Model file for the job. Use its own axes, mm. A direction names the side the tool comes from. Round coordinates to 2 decimals unless told otherwise and drop trailing zeros. Loops run counter-clockwise (first coordinate to the right, second up) from the corner with the lowest first, then second, coordinate; pieces in that order, holes last. Notation, with made-up numbers: (-33.75, -21) -> (13.25, -21) arc R6 ccw to (13.25, -12) -> close; hole circle Ø7 at (1.5, -36). An arc over 180 degrees is marked (long way). Use a Markdown table: item, result. Add a question column.
Autodesk Inventor part; units mm, degrees
ref_plane "YZ Plane" through (0, 0, 0) normal (1, 0, 0) x (0, 1, 0)
ref_plane "XZ Plane" through (0, 0, 0) normal (0, 1, 0) x (-1, 0, 0)
ref_plane "XY Plane" through (0, 0, 0) normal (0, 0, 1) x (1, 0, 0)
sketch "Sketch1" plane through (0, 0, 0) normal (0, 1, 0) x (-1, 0, 0)
  arc A0 (-0.3814, 2.9757) -> (-3, 0) centre (0, 0) ccw
  arc A1 (-0.3814, 2.9757) -> (0, 75) centre (-5, 39.0133) ccw
  line L0 (-105, 0) -> (0, 0) construction
  line L1 (-3, 0) -> (-105, 0) construction
  arc A2 (-3, 0) -> (-0.3814, -2.9757) centre (0, 0) ccw
  arc A3 (-1.6619, -2.4976) -> (97.0992, -0.9275) centre (46.5785, 70) ccw
  arc A4 (102.9008, -9.0725) -> (97.0992, -0.9275) centre (100, -5) ccw
  line L2 (0, 0) -> (100, 0) construction
  arc A5 (5.6849, -18.0476) -> (102.9008, -9.0725) centre (46.5785, 70) ccw
  line L3 (0, 75) -> (0, 0) construction
  line L4 (0, 0) -> (0, -15.1769) construction
  line L5 (0, 0) -> (-105, 0) construction
  line L6 (0, 75) -> (-105, 75)
  line L7 (-105, 75) -> (-105, -25)
  line L8 (0, -21.6754) -> (0, -21)
  line L9 (-4, -25) -> (-105, -25)
  arc A6 (5.6849, -18.0476) -> (0, -21.6754) centre (4, -21.6754) ccw
  arc A7 (-4, -25) -> (0, -21) centre (-4, -21) ccw
  circle A8 centre (-5, 35) radius 11
  point P0 (-5, -39.0133)
  point P1 (0, -25)
  dimension "d0" = 6
  dimension "d13" = 5
  dimension "d47" = 10
  dimension "d48" = 100
  dimension "d49" = 100
  dimension "d68" = 70
  dimension "d71" = 0
  dimension "d73" = 25
  dimension "d75" = 105
  dimension "d76" = 4
  dimension "d77" = 4
  dimension "d101" = 22
  dimension "d102" = 5
  dimension "d103" = 35
  dimension "d108" = 75
extrude "Extrusion1" add sketch "Sketch1" along normal blind 2
sketch "Szkic5" plane through (0, 2, 0) normal (0, 1, 0) x (1, 0, 0)
  circle A0 centre (12.5, -67.5) radius 2.1
  circle A1 centre (97.5, -67.5) radius 2.1
  line L0 (97.5, -67.5) -> (97.5, 52.5) construction
  line L1 (12.5, -67.5) -> (97.5, -67.5) construction
  line L2 (0, -75) -> (105, -75) construction
  line L3 (105, -75) -> (105, 25) construction
  line L4 (105, 25) -> (4, 25) construction
  line L5 (0, 21) -> (0, 21.6754) construction
  circle A2 centre (97.5, 20) radius 2.1
  circle A3 centre (12.5, 20) radius 2.1
  line L6 (12.5, 20) -> (97.5, 20) construction
  point P0 (0, 0)
  dimension "d84" = 7.5
  dimension "d85" = 7.5
  dimension "d89" = 85
  dimension "d106" = 87.5
  dimension "d107" = 85
  dimension "d109" = 4.2
extrude "Wyciągnięcie proste4" cut sketch "Szkic5" against normal up to surface (2 mm away)
sketch "Szkic6" plane through (0, 2, 0) normal (0, 1, 0) x (1, 0, 0)
  line L0 (105, -55) -> (100.9, -55)
  line L1 (100.9, -55) -> (100.9, -40)
  line L2 (100.9, -40) -> (105, -40)
  line L3 (105, -40) -> (105, -55)
  line L4 (105, -10) -> (100.9, -10)
  line L5 (100.9, -10) -> (100.9, 5)
  line L6 (100.9, 5) -> (105, 5)
  line L7 (105, 5) -> (105, -10)
  line L8 (100.9, -40) -> (100.9, -10) construction
  line L9 (105, -75) -> (105, 25) construction
  line L10 (100.9, -25) -> (105, -25) construction
  point P0 (0, 0)
  dimension "d92" = 15
  dimension "d94" = 30
  dimension "d134" = 4.1
extrude "Wyciągnięcie proste5" cut sketch "Szkic6" against normal up to surface (2 mm away)
sketch "Sketch9" plane through (0, 2, 0) normal (0, 1, 0) x (1, 0, 0)
  line L0 (-11.5, -35) -> (21.5, -35) construction
  circle A0 centre (-11.5, -35) radius 1.6
  circle A1 centre (21.5, -35) radius 1.6
  circle A2 centre (5, -35) radius 11 construction
  point P0 (0, 0)
  dimension "d110" = 33
  dimension "d111" = 3.2
extrude "Extrusion6" cut sketch "Sketch9" against normal through all
fillet "Fillet1" radius 5 1 edges at (105, 1, -25)
sketch "Sketch10" plane through (0, 2, 0) normal (0, 1, 0) x (1, 0, 0)
  circle A0 centre (6, 12.5) radius 1.75
  circle A1 centre (34, 12.5) radius 1.75
  line L0 (6, 12.5) -> (34, 12.5) construction
  line L1 (100, 25) -> (4, 25) construction
  point P0 (0, 0)
  dimension "d115" = 3.5
  dimension "d116" = 28
  dimension "d117" = 12.5
  dimension "d118" = 6
extrude "Extrusion7" cut sketch "Sketch10" against normal through all
sketch "Sketch11" plane through (0, 2, 0) normal (0, 1, 0) x (1, 0, 0)
  line L0 (93.5, -75) -> (51.5, -75)
  line L1 (51.5, -75) -> (51.5, -18)
  line L2 (51.5, -18) -> (93.5, -18)
  line L3 (93.5, -18) -> (93.5, -75)
  line L4 (0, -75) -> (105, -75) construction
  point P0 (0, 0)
  point P1 (100, -75)
  dimension "d121" = 42
  dimension "d122" = 57
  dimension "d123" = 51.5
extrude "Extrusion8" cut sketch "Sketch11" against normal through all
sketch "Sketch12" plane through (0, 2, 0) normal (0, 1, 0) x (1, 0, 0)
  line L0 (93.5, -75) -> (105, -75)
  line L1 (93.5, -75) -> (93.5, -90.5)
  line L2 (93.5, -90.5) -> (51.5, -90.5)
  line L3 (0, -75) -> (51.5, -75)
  line L4 (51.5, -90.5) -> (51.5, -75)
  line L5 (93.5, -75) -> (105, -75)
  line L6 (105, -75) -> (105, -98.5)
  line L7 (105, -98.5) -> (43.5, -98.5)
  line L8 (43.5, -98.5) -> (43.5, -75)
  point P0 (0, 0)
  dimension "d126" = 15.5
  dimension "d127" = 8
  dimension "d128" = 8
extrude "Extrusion9" add sketch "Sketch12" against normal up to surface (2 mm away)
fillet "Fillet2" radius 5 3 edges at (43.5, 1, 75) (43.5, 1, 98.5) (105, 1, 98.5)
fillet "Fillet3" radius 1 4 edges at (51.5, 1, 18) (93.5, 1, 18) (93.5, 1, 90.5) (51.5, 1, 90.5)
fillet "Fillet4" radius 2 4 edges at (105, 1, 55) (105, 1, 40) (105, 1, 10) (105, 1, -5)
sketch "Sketch13" plane through (0, 2, 0) normal (0, 1, 0) x (1, 0, 0)
  line L0 (99.25, -77.5) -> (99.25, -93.5) construction
  line L1 (93.5, -19) -> (93.5, -89.5) construction
  line L2 (93.5, -89.5) -> (105, -89.5) construction
  line L3 (105, -93.5) -> (105, -57) construction
  point P0 (0, 0)
  point P1 (99.25, -89.5)
  dimension "d137" = 12
  dimension "d138" = 4
hole "Hole1" at (99.25, 2, 77.5) at (99.25, 2, 93.5) direction (0, -1, 0) diameter 3.2 end through all
sketch "Sketch14" plane through (0, 2, 0) normal (0, 1, 0) x (1, 0, 0)
  arc A0 (1.6619, 2.4976) -> (-97.0992, 0.9275) centre (-46.5785, -70) ccw construction
  arc A1 (-102.9008, 9.0725) -> (-97.0992, 0.9275) centre (-100, 5) ccw
  arc A2 (13.245, 0) -> (-100, 5) centre (-46.5785, -70) ccw construction
  line L0 (0, 0) -> (13.245, 0) construction
  line L1 (-46.5785, -70) -> (-100, 5) construction
  line L2 (24.9599, 21) -> (84.9599, 21) construction
  circle A3 centre (12.5, 20) radius 2.1
  circle A4 centre (97.5, 20) radius 2.1
  line L3 (100, 25) -> (4, 25)
  line L4 (0, -70) -> (38.5, -70) construction
  arc A5 (43.5, -80) -> (38.5, -75) centre (38.5, -80) ccw
  line L5 (38.5, -70) -> (38.5, -75) construction
  line L6 (0, -75) -> (0, -70) construction
  line L7 (0, -75) -> (38.5, -75)
  arc A6 (100, -98.5) -> (105, -93.5) centre (100, -93.5) ccw
  line L8 (48.5, -93.5) -> (100, -93.5) construction
  arc A7 (43.5, -93.5) -> (48.5, -98.5) centre (48.5, -93.5) ccw construction
  arc A8 (100, -98.5) -> (105, -93.5) centre (100, -93.5) ccw construction
  point P0 (54.9599, 21)
  point P1 (74.25, -93.5)
  point P2 (-78.7683, 16.2709)
  point P3 (-78.7683, 16.2709)
  point P4 (-78.7683, 16.2709)
  point P5 (-55.3429, 21.6626)
  point P6 (-55.3429, 21.6626)
  point P7 (-55.3429, 21.6626)
  point P8 (-31.3202, 20.8077)
  point P9 (-31.3202, 20.8077)
  point P10 (-31.3202, 20.8077)
  point P11 (-8.3374, 13.7643)
  point P12 (-8.3374, 13.7643)
  point P13 (-8.3374, 13.7643)
  dimension "d150" = 60
  dimension "d151" = 12.5
  dimension "d152" = 4
  dimension "d153" = 5
  dimension "d156" = 60
hole "Hole2" at (-100, 2, -5) at (24.9599, 2, -21) at (54.9599, 2, -21) at (84.9599, 2, -21) at (0, 2, 70) at (38.5, 2, 70) at (48.5, 2, 93.5) at (74.25, 2, 93.5) at (-78.7683, 2, -16.2709) at (-55.3429, 2, -21.6626) at (-31.3202, 2, -20.8077) at (-8.3374, 2, -13.7643) direction (0, -1, 0) diameter 3.2 end through all
sketch "Sketch15" plane through (0, 2, 0) normal (0, 1, 0) x (1, 0, 0)
  line L0 (30, -40) -> (31.5, -40)
  line L1 (31.5, -40) -> (31.5, -51)
  line L2 (31.5, -51) -> (30, -51)
  line L3 (30, -51) -> (30, -40)
  line L4 (41.5, -40) -> (43, -40)
  line L5 (43, -40) -> (43, -51)
  line L6 (43, -51) -> (41.5, -51)
  line L7 (41.5, -51) -> (41.5, -40)
  point P0 (0, 0)
  dimension "d165" = 1.5
  dimension "d166" = 11
  dimension "d167" = 10
  dimension "d168" = 40
  dimension "d169" = 30
extrude "Extrusion10" cut sketch "Sketch15" against normal through all
sketch "Sketch16" plane through (0, 2, 0) normal (0, 1, 0) x (1, 0, 0)
  line L0 (43, -40) -> (43, -51)
  line L1 (43, -51) -> (41.5, -51)
  line L2 (41.5, -51) -> (41.5, -40)
  line L3 (41.5, -40) -> (43, -40)
  line L4 (31.5, -40) -> (31.5, -51)
  line L5 (31.5, -51) -> (30, -51)
  line L6 (30, -51) -> (30, -40)
  line L7 (30, -40) -> (31.5, -40)
  circle A0 centre (-31.3202, 20.8077) radius 1.6
  circle A1 centre (-78.7683, 16.2709) radius 1.6
  circle A2 centre (48.5, -93.5) radius 1.6
  circle A3 centre (0, -70) radius 1.6
  circle A4 centre (54.9599, 21) radius 1.6
  circle A5 centre (-100, 5) radius 1.6
  circle A6 centre (24.9599, 21) radius 1.6
  circle A7 centre (84.9599, 21) radius 1.6
  circle A8 centre (38.5, -70) radius 1.6
  circle A9 centre (74.25, -93.5) radius 1.6
  circle A10 centre (-55.3429, 21.6626) radius 1.6
  circle A11 centre (-8.3374, 13.7643) radius 1.6
  circle A12 centre (99.25, -77.5) radius 1.6
  circle A13 centre (99.25, -93.5) radius 1.6
  line L8 (51.5, -89.5) -> (51.5, -19)
  arc A14 (52.5, -18) -> (51.5, -19) centre (52.5, -19) ccw
  line L9 (52.5, -18) -> (92.5, -18)
  arc A15 (93.5, -19) -> (92.5, -18) centre (92.5, -19) ccw
  line L10 (93.5, -19) -> (93.5, -89.5)
  arc A16 (92.5, -90.5) -> (93.5, -89.5) centre (92.5, -89.5) ccw
  line L11 (92.5, -90.5) -> (52.5, -90.5)
  arc A17 (51.5, -89.5) -> (52.5, -90.5) centre (52.5, -89.5) ccw
  circle A18 centre (34, 12.5) radius 1.75
  circle A19 centre (6, 12.5) radius 1.75
  circle A20 centre (-11.5, -35) radius 1.6
  circle A21 centre (21.5, -35) radius 1.6
  circle A22 centre (97.5, 20) radius 2.1
  circle A23 centre (12.5, 20) radius 2.1
  circle A24 centre (97.5, -67.5) radius 2.1
  circle A25 centre (12.5, -67.5) radius 2.1
  circle A26 centre (5, -35) radius 11
  arc A27 (103, 5) -> (105, 7) centre (103, 7) ccw
  line L12 (105, 7) -> (105, 20)
  arc A28 (105, 20) -> (100, 25) centre (100, 20) ccw
  line L13 (100, 25) -> (4, 25)
  arc A29 (4, 25) -> (0, 21) centre (4, 21) ccw
  line L14 (0, 21) -> (0, 21.6754)
  arc A30 (-5.6849, 18.0476) -> (0, 21.6754) centre (-4, 21.6754) ccw
  arc A31 (-5.6849, 18.0476) -> (-102.9008, 9.0725) centre (-46.5785, -70) ccw
  arc A32 (-102.9008, 9.0725) -> (-97.0992, 0.9275) centre (-100, 5) ccw
  arc A33 (1.6619, 2.4976) -> (-97.0992, 0.9275) centre (-46.5785, -70) ccw
  arc A34 (0.3814, -2.9757) -> (1.6619, 2.4976) centre (0, 0) ccw
  arc A35 (0.3814, -2.9757) -> (0, -75) centre (5, -39.0133) ccw
  line L15 (0, -75) -> (38.5, -75)
  arc A36 (43.5, -80) -> (38.5, -75) centre (38.5, -80) ccw
  line L16 (43.5, -80) -> (43.5, -93.5)
  arc A37 (43.5, -93.5) -> (48.5, -98.5) centre (48.5, -93.5) ccw
  line L17 (48.5, -98.5) -> (100, -98.5)
  arc A38 (100, -98.5) -> (105, -93.5) centre (100, -93.5) ccw
  line L18 (105, -93.5) -> (105, -57)
  arc A39 (105, -57) -> (103, -55) centre (103, -57) ccw
  line L19 (103, -55) -> (100.9, -55)
  line L20 (100.9, -55) -> (100.9, -40)
  line L21 (100.9, -40) -> (103, -40)
  arc A40 (103, -40) -> (105, -38) centre (103, -38) ccw
  line L22 (105, -38) -> (105, -12)
  arc A41 (105, -12) -> (103, -10) centre (103, -12) ccw
  line L23 (103, -10) -> (100.9, -10)
  line L24 (100.9, -10) -> (100.9, 5)
  line L25 (100.9, 5) -> (103, 5)
  point P0 (0, 0)
  dimension "d172" = 10
  dimension "d173" = 1.75
properties part number "wstepna_geometria_wersja_2" material "Aluminum 6061"
1) Cut at A-A on x = 63.5. Write the cut outline in (y, z).
2) Cut at C-C on z = 5. Write the cut outline in (x, y), and give its area (3 significant figures).
3) Pin check, flat tips, straight feed: pin 1 Ø0.6 at (y, z) = (0.5, 59) entering from -X; pin 2 Ø0.6 at (x, y) = (102, 1) entering from +Z; pin 3 Ø0.8 at (x, y) = (30.5, 1.5) entering from +Z. Stop position of each tip, or through.
4) Pull direction Z, two halves, no side cores. Call faces 1 (the face through (22, 2, 21)), 2 (the face through (-31.33, 0.99, 39.55)), 3 (the face through (-1.801, 0.986, -18.334)): +Z half, -Z half, draft (parallel to the pull), parting line (faces both ways), or undercut.
5) Tool access for faces 4 (the face through (-48.698, 0.986, -17.055)), 5 (the face through (45, 0.99, 97.07)): list every direction of +Z, -Z, +X, -X, +Y, -Y with a clear straight run to the whole face (end or side of a thin tool).
6) Cut at D-D on y = 1.6. Count the separate pieces of the cut face and the enclosed holes in it, and give its area (3 significant figures).
7) Cut at B-B on z = 48.5. Write the cut outline in (x, y), and give its area (3 significant figures).
8) Wall check: probe 1 along Z at (x, y) = (97.5, 0.4); probe 2 along Z at (x, y) = (74.25, 1.6); probe 3 along X at (y, z) = (0.6, 93.5). Give the ranges that are in metal, low to high. Write a range as from..to.
Established:
| question | item | result |
|---|---|---|
| 1 | outline | (0, -25) -> (2, -25) -> (2, 18) -> (0, 18) -> close; (0, 90.5) -> (2, 90.5) -> (2, 98.5) -> (0, 98.5) -> close |
| 2 | outline | (-7.77, 0) -> (100.9, 0) -> (100.9, 2) -> (-7.77, 2) -> close |
| 2 | area | 217 mm^2 |
| 3 | pin 1 | stops at x = -25.54 |
| 3 | pin 2 | stops at z = 98.2 |
| 3 | pin 3 | stops at z = 75 |
| 4 | face 1 | draft |
| 4 | face 2 | undercut |
| 4 | face 3 | -Z half |
| 5 | face 4 | +Y, -Y |
| 5 | face 5 | +Z, -X, +Y, -Y |
| 6 | separate pieces | 1 |
| 6 | enclosed holes | 26 |
| 6 | area | 10,900 mm^2 |
| 7 | outline | (-30.07, 0) -> (30, 0) -> (30, 2) -> (-30.07, 2) -> close; (31.5, 0) -> (41.5, 0) -> (41.5, 2) -> (31.5, 2) -> close; (43, 0) -> (51.5, 0) -> (51.5, 2) -> (43, 2) -> close; (93.5, 0) -> (100.9, 0) -> (100.9, 2) -> (93.5, 2) -> close |
| 7 | area | 172 mm^2 |
| 8 | probe 1 | z = -25..-22.1, -17.9..65.4, 69.6..98.5 |
| 8 | probe 2 | z = -25..18, 90.5..91.9, 95.1..98.5 |
| 8 | probe 3 | x = 43.5..46.9, 50.1..72.65, 75.85..97.65, 100.85..105 |
